Can you work these out from the model? Positions are in its coordinate system, mm. A direction names the side the tool comes from. Coordinates: 2 decimals unless noted, no trailing zeros. Loops run counter-clockwise (first coordinate to the right, second up) from the corner with the lowest first, then second, coordinate; pieces in that order, holes last. Notation, with made-up numbers: (-17.5, -12.5) -> (-4.5, -12.5) arc R20 cw to (-4.5, 26.5) -> close; hole circle Ø10 at (68.25, 47.25). An arc over 180 degrees is marked (long way). Use one line per item in the form item = value. Start each with the question number.
(1) I need wall thicknesses on line 1 (X direction, y = -4.1, z = 40.5); line 2 (Z direction, x = 26, y = -0.8); line 3 (X direction, y = -3.9, z = 28.5). Which ranges of each line are inside material? Lowest first, please. Write a range as [from, to].
(2) I'm going to push flat-ended pins straight in: pin 1 (10 mm diameter, centred on x = 12, z = 30.5, fed in from +Y); pin 2 (3 mm diameter, centred on x = 12, y = -2.5, fed in from +Z); pin 3 (1.5 mm diameter, centred on x = 15, y = -2.5, fed in from -Z). Where does each tip first touch, or does it pass through?
(3) Imagine slicing it at B-B (z = 24). List the corners of the cut face in (x, y) for me, plus the area to 3 significant figures.
(4) Imagine slicing it at A-A (x = -15.5). List the corners of the cut face in (y, z) for me.
(5) On a 3-axis mill with a long thin cutter (end or side, diameter ignored), from which of +Z, -Z, +X, -X, +Y, -Y can I reach the whole of each face in a straight line? I mean faces 5 (the flat face through (-30.842, -3, -14)), 6 (the flat face through (-25, -3, -45.842)), 7 (the flat face through (-25, -3, 28)), 8 (the flat face through (-6.667, -3, 43)), 9 (the flat face through (28, -3, 21)). Say none if no direction works.
(6) Thinking about a two-plate mould opening in Z: for faces 1 (the flat face through (25, -3, -28)), 2 (the flat face through (0, -5.842, 1)), 3 (the flat face through (28, -3, -21)), 4 (the flat face through (-13, -3, -40)), which applies, released by +Z, released by -Z, zero draft, split by the parting line, or undercut?
```python
from build123d import *

# Parameters (mm, degrees)
F1_DEPTH = 5.842


with BuildPart() as f1:
    # F0 (on Front) → F1 (new body)
    with BuildSketch(Plane.XZ):
        Polygon((-20, -45.842), (-20, -40), (-6.666667, -40), (-6.666667, -45.842), (6.666667, -45.842), (6.666667, -40), (20, -40), (20, -45.842), (30.842, -45.842), (30.842, -35), (25, -35), (25, -21), (30.842, -21), (30.842, -7), (25, -7), (25, 7), (30.842, 7), (30.842, 21), (25, 21), (25, 35), (30.842, 35), (30.842, 45.842), (20, 45.842), (20, 40), (6.666667, 40), (6.666667, 45.842), (-6.666667, 45.842), (-6.666667, 40), (-20, 40), (-20, 45.842), (-30.842, 45.842), (-30.842, 35), (-25, 35), (-25, 21), (-30.842, 21), (-30.842, 7), (-25, 7), (-25, -7), (-30.842, -7), (-30.842, -21), (-25, -21), (-25, -35), (-30.842, -35), (-30.842, -45.842), align=None)
    extrude(amount=F1_DEPTH)


solid = f1.part
```
Worked out:
q1.line_1 = [-30.84, -20], [-6.67, 6.67], [20, 30.84]
q1.line_2 = [-45.84, -35], [-21, -7], [7, 21], [35, 45.84]
q1.line_3 = [-25, 25]
q2.pin_1 = 0
q2.pin_2 = 40
q2.pin_3 = -40
q3.outline = (-25, -5.84) -> (25, -5.84) -> (25, 0) -> (-25, 0) -> close
q3.area = 292 mm2
q4.outline = (-5.84, -40) -> (0, -40) -> (0, 40) -> (-5.84, 40) -> close
q5.face_5 = +Z, -Z, -X, +Y, -Y
q5.face_6 = -Z, +X, -X, +Y, -Y
q5.face_7 = -X, +Y, -Y
q5.face_8 = +Z, +Y, -Y
q5.face_9 = +X, +Y, -Y
q6.face_1 = undercut
q6.face_2 = zero draft
q6.face_3 = undercut
q6.face_4 = released by -Z
